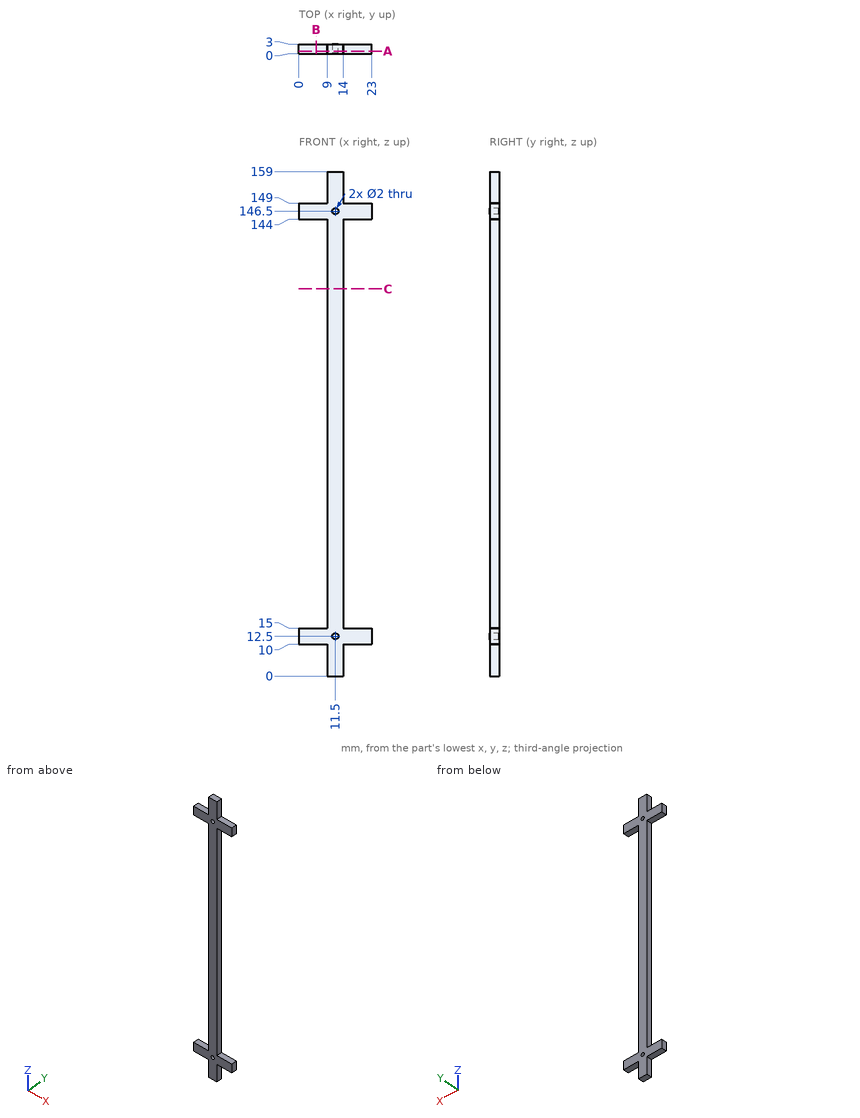
Geometry check sheet. Reference: drawing and pictorial views, mm from the part's lowest x, y, z. Give positions to 0.01 mm unless a question says otherwise; leave off trailing zeros. Write each loop counter-clockwise with the first axis right and the second up, starting at its lowest first coordinate (ties: lowest second). Pieces come first, ordered by that corner, then holes. Notation, with made-up numbers: (10, 43.25) -> (27, 43.25) arc R15 cw to (27, 72.25) -> close; hole circle Ø1 at (58.5, 9.5). An arc over 180 degrees is marked (long way). One line per item, written item: value. Start each with the question number.
Item 1: Gauge pin test, flat ends, axial feed: pin 1 (0.9 mm diameter, centred on x = 6, y = 1.5, fed in from +Z); pin 2 (1.5 mm diameter, centred on y = 1, z = 153, fed in from -X); pin 3 (1.5 mm diameter, centred on y = 1, z = 28.5, fed in from +X); pin 4 (1.6 mm diameter, centred on x = 11.5, z = 12.5, fed in from -Y). Record the tip position at first contact, or that the pin passes through.
Item 2: Section check B-B on x = 5.5. Record the cut outline in (y, z).
Item 3: Material ranges on probe 1 along Z at (x, y) = (11.5, 1.4); probe 2 along Z at (x, y) = (1.5, 1.6); probe 3 along X at (y, z) = (1.05, 12.5), recorded low to high. Write a range as from..to.
Item 4: Section check A-A on y = 0.75. Record the cut outline in (x, z).
Item 5: Section check C-C on z = 122. Record the cut outline in (x, y), then the cut area to 3 significant figures.
Results list:
1. pin 1: z = 149
1. pin 2: x = 9
1. pin 3: x = 14
1. pin 4: through
2. outline: (0, 10) -> (3, 10) -> (3, 15) -> (0, 15) -> close; (0, 144) -> (3, 144) -> (3, 149) -> (0, 149) -> close
3. probe 1: 0..11.5, 13.5..145.5, 147.5..159
3. probe 2: 10..15, 144..149
3. probe 3: 0..10.5, 12.5..23
4. outline: (0, 10) -> (9, 10) -> (9, 0) -> (14, 0) -> (14, 10) -> (23, 10) -> (23, 15) -> (14, 15) -> (14, 144) -> (23, 144) -> (23, 149) -> (14, 149) -> (14, 159) -> (9, 159) -> (9, 149) -> (0, 149) -> (0, 144) -> (9, 144) -> (9, 15) -> (0, 15) -> close; hole circle Ø2 at (11.5, 12.5); hole circle Ø2 at (11.5, 146.5)
5. outline: (9, 0) -> (14, 0) -> (14, 3) -> (9, 3) -> close
5. area: 15.0 mm²
